from build123d import *

# Parameters (mm, degrees)
F0_W     = 1215.898
F0_H     = 2435.098
F1_DEPTH = 14.3002
F2_W     = 12.7
F2_H     = 2435.098
F3_DEPTH = 12.7


# Not quite as in the source:
# - a feature names something its author has since deleted; it is built from what else it names


with BuildPart() as f1:
    # F0 (on Right) → F1 (new body)
    with BuildSketch(Plane.YZ):
        with Locations((607.949, 1217.549)):
            Rectangle(F0_W, F0_H)
    extrude(amount=F1_DEPTH)

    # F2 (on face) → F3 (join)
    with BuildSketch(Plane.YZ.offset(14.3002)):
        with Locations((425.45, 1217.549)):
            Rectangle(F2_W, F2_H)
        with Locations((641.35, 1217.549)):
            Rectangle(F2_W, F2_H)
        with Locations((857.25, 1217.549)):
            Rectangle(F2_W, F2_H)
        with Locations((1073.15, 1217.549)):
            Rectangle(F2_W, F2_H)
        with Locations((209.55, 1217.549)):
            Rectangle(F2_W, F2_H)
    extrude(amount=F3_DEPTH)


solid = f1.part
The model under review builds one solid part; all positions refer to its coordinate system, in mm. A direction names the side the tool comes from. Coordinates: 2 decimals unless noted, no trailing zeros. Loops run counter-clockwise (first coordinate to the right, second up) from the corner with the lowest first, then second, coordinate; pieces in that order, holes last.
(1) Consider section A-A, the plane z = 269. Give the boundary of the cut face in (x, y), plus the area to 3 significant figures.
Determined:
outline: (0, 0) - (14.3, 0) - (14.3, 203.2) - (27, 203.2) - (27, 215.9) - (14.3, 215.9) - (14.3, 419.1) - (27, 419.1) - (27, 431.8) - (14.3, 431.8) - (14.3, 635) - (27, 635) - (27, 647.7) - (14.3, 647.7) - (14.3, 850.9) - (27, 850.9) - (27, 863.6) - (14.3, 863.6) - (14.3, 1066.8) - (27, 1066.8) - (27, 1079.5) - (14.3, 1079.5) - (14.3, 1215.9) - (0, 1215.9) - close
area: 18,200 mm2
(2) Consider section B-B, the plane y = 1013.5. Give the boundary of the cut face in (x, z).
Determined:
outline: (0, 0) - (14.3, 0) - (14.3, 2435.1) - (0, 2435.1) - close
(3) Draft analysis for pull direction Y (two halves, no side actions). For faces 1 (the flat face through (14.3, 964, 1235)), 2 (the flat face through (0, 599, 1235)), state which applies: +Y half, -Y half, draft (parallel to the pull), parting line (faces both ways), or undercut.
Determined:
face 1: undercut
face 2: draft
(4) Tool access review of faces 3 (the flat face through (14.3, 532, 1235)), 4 (the flat face through (14.3, 100, 1235)), 5 (the flat face through (14.3, 1147, 1235)): name each direction out of +Z, -Z, +X, -X, +Y, -Y from which nothing blocks a thin tool from reaching the whole face with its end or side.
Determined:
face 3: +Z, -Z, +X
face 4: +Z, -Z, +X, -Y
face 5: +Z, -Z, +X, +Y
(5) Wall thickness on L1, parallel to Y at x = 18, z = 984; L2, parallel to X at y = 520.5, z = 2336: over which ranges is each line inside the solid? List them lowest first.
Determined:
L1: y = 203.2 to 215.9, 419.1 to 431.8, 635 to 647.7, 850.9 to 863.6, 1066.8 to 1079.5
L2: x = 0 to 14.3
(6) Insertion check: P1, Ø2, axis at y = 871.5, z = 1626.5, coming from the +X side; P2, Ø4, axis at x = 23.5, z = 1243.5, coming from the +Y side; P3, Ø4, axis at x = 22, z = 1687.5, coming from the -Y side. Each pin has a flat end and moves straight along its axis. Give the tip position at first contact, or say it passes through.
Determined:
P1: stops at x = 14.3
P2: stops at y = 1079.5
P3: stops at y = 203.2
